```python
from build123d import *

# Parameters (mm, degrees)
BOSS_EXTRUDE1_DEPTH     = 16
F_8_0MM_DOWEL_HOLE1_D   = 8
CIRPATTERN2_COUNT       = 5
CIRPATTERN2_ANGLE       = 180
MIRROR2_COPY_1_D        = 8
MIRROR2_COPY_2_D        = 8
MIRROR2_COPY_3_D        = 8
MIRROR2_COPY_4_D        = 8
LPATTERN1_COUNT         = 3
LPATTERN1_PITCH         = 74
MIRROR3_COPY_1_D        = 8
MIRROR3_COPY_2_D        = 8
MIRROR3_COPY_3_D        = 8
SKETCH13_R              = 4
SKETCH13_R_2            = 10
BOSS_EXTRUDE2_DEPTH     = 16
BOSS_EXTRUDE3_DEPTH     = 26
SKETCH16_W              = 10
SKETCH16_H              = 10
BOSS_EXTRUDE5_DEPTH     = 5
M10X1_25_TAPPED_HOLE1_D = 8.8
SKETCH19_R              = 16
CUT_EXTRUDE1_DEPTH      = 32


with BuildPart() as part:
    # Sketch1 → Boss-Extrude1 (new body)
    with BuildSketch(Plane(origin=(0, 0, 0), x_dir=(1, 0, 0), z_dir=(0, 1, 0))):
        with BuildLine():
            Line((-110, 110), (110, 110))
            ThreePointArc((110, 110), (220, 0), (110, -110))
            Line((110, -110), (-110, -110))
            ThreePointArc((-110, -110), (-220, 0), (-110, 110))
        make_face()
        with BuildLine():
            Line((-110, 90), (110, 90))
            ThreePointArc((110, 90), (200, 0), (110, -90))
            Line((110, -90), (-110, -90))
            ThreePointArc((-110, -90), (-200, 0), (-110, 90))
        make_face(mode=Mode.SUBTRACT)
    extrude(amount=BOSS_EXTRUDE1_DEPTH)

    # Ø8.0mm Dowel Hole1 (through all)
    with Locations(Plane(origin=(-110, 16, -100), x_dir=(0, 0, 1), z_dir=(0, 1, 0))):
        with Locations((0, 0)):
            f_8_0mm_dowel_hole1 = Hole(F_8_0MM_DOWEL_HOLE1_D / 2)

    # CirPattern2: Ø8.0mm Dowel Hole1 ×5 about axis
    cirpattern2_axis = Axis((-110, 0, 0), (0, 1, 0))
    for i in range(1, CIRPATTERN2_COUNT):
        add(f_8_0mm_dowel_hole1.rotate(cirpattern2_axis, i * CIRPATTERN2_ANGLE / (CIRPATTERN2_COUNT - 1)), mode=Mode.SUBTRACT)

    # Mirror2: Ø8.0mm Dowel Hole1 across plane
    add(f_8_0mm_dowel_hole1.mirror(Plane(origin=(0, 0, 0), x_dir=(0, 0, 1), z_dir=(1, 0, 0))), mode=Mode.SUBTRACT)

    # Mirror2 copy 1 (through all)
    with Locations(Plane(origin=(180.710678119, 16, -70.710678119), x_dir=(-0.707106781, 0, 0.707106781), z_dir=(0, 1, 0))):
        with Locations((0, 0)):
            Hole(MIRROR2_COPY_1_D / 2)

    # Mirror2 copy 2 (through all)
    with Locations(Plane(origin=(210, 16, 0), x_dir=(-1, 0, 0), z_dir=(0, 1, 0))):
        with Locations((0, 0)):
            Hole(MIRROR2_COPY_2_D / 2)

    # Mirror2 copy 3 (through all)
    with Locations(Plane(origin=(180.710678119, 16, 70.710678119), x_dir=(-0.707106781, 0, -0.707106781), z_dir=(0, 1, 0))):
        with Locations((0, 0)):
            Hole(MIRROR2_COPY_3_D / 2)

    # Mirror2 copy 4 (through all)
    with Locations(Plane(origin=(110, 16, 100), x_dir=(0, 0, -1), z_dir=(0, 1, 0))):
        with Locations((0, 0)):
            Hole(MIRROR2_COPY_4_D / 2)

    # LPattern1: Ø8.0mm Dowel Hole1 ×3
    with Locations(*[(i * LPATTERN1_PITCH, 0, 0) for i in range(1, LPATTERN1_COUNT)]):
        add(f_8_0mm_dowel_hole1, mode=Mode.SUBTRACT)

    # Mirror3 copy 1 (through all)
    with Locations(Plane(origin=(-36, 16, 100), x_dir=(0, 0, -1), z_dir=(0, 1, 0))):
        with Locations((0, 0)):
            Hole(MIRROR3_COPY_1_D / 2)

    # Mirror3 copy 2 (through all)
    with Locations(Plane(origin=(38, 16, 100), x_dir=(0, 0, -1), z_dir=(0, 1, 0))):
        with Locations((0, 0)):
            Hole(MIRROR3_COPY_2_D / 2)

    # Mirror3 copy 3 (through all)
    with Locations(Plane(origin=(-110, 16, 100), x_dir=(0, 0, -1), z_dir=(0, 1, 0))):
        with Locations((0, 0)):
            Hole(MIRROR3_COPY_3_D / 2)

    # Sketch13 → Boss-Extrude2 (add)
    with BuildSketch(Plane(origin=(0, 0, 0), x_dir=(1, 0, 0), z_dir=(0, 1, 0))):
        with BuildLine():
            Line((-110, -110), (110, -110))
            ThreePointArc((110, -110), (220, 0), (110, 110))
            Line((110, 110), (-110, 110))
            ThreePointArc((-110, 110), (-220, 0), (-110, -110))
        make_face()
        with Locations((38, -100)):
            Circle(SKETCH13_R, mode=Mode.SUBTRACT)
        with Locations((-110, 100)):
            Circle(SKETCH13_R, mode=Mode.SUBTRACT)
        with Locations((-180.710678119, 70.710678119)):
            Circle(SKETCH13_R, mode=Mode.SUBTRACT)
        with Locations((-210, 0)):
            Circle(SKETCH13_R, mode=Mode.SUBTRACT)
        with Locations((-180.710678119, -70.710678119)):
            Circle(SKETCH13_R, mode=Mode.SUBTRACT)
        with Locations((-110, -100)):
            Circle(SKETCH13_R, mode=Mode.SUBTRACT)
        with Locations((110, 100)):
            Circle(SKETCH13_R, mode=Mode.SUBTRACT)
        with Locations((180.710678119, 70.710678119)):
            Circle(SKETCH13_R, mode=Mode.SUBTRACT)
        with Locations((210, 0)):
            Circle(SKETCH13_R, mode=Mode.SUBTRACT)
        with Locations((180.710678119, -70.710678119)):
            Circle(SKETCH13_R, mode=Mode.SUBTRACT)
        with Locations((110, -100)):
            Circle(SKETCH13_R, mode=Mode.SUBTRACT)
        with Locations((-36, 100)):
            Circle(SKETCH13_R, mode=Mode.SUBTRACT)
        with Locations((38, 100)):
            Circle(SKETCH13_R, mode=Mode.SUBTRACT)
        with Locations((-36, -100)):
            Circle(SKETCH13_R, mode=Mode.SUBTRACT)
        with Locations((-165, -50)):
            Circle(SKETCH13_R_2, mode=Mode.SUBTRACT)
        with Locations((-165, 50)):
            Circle(SKETCH13_R_2, mode=Mode.SUBTRACT)
    extrude(amount=BOSS_EXTRUDE2_DEPTH)

    # Sketch15 → Boss-Extrude3 (add)
    with BuildSketch(Plane(origin=(0, 0, 0), x_dir=(1, 0, 0), z_dir=(0, 1, 0))):
        with BuildLine():
            ThreePointArc((-130, 70), (-124.142135624, 84.142135624), (-110, 90))
            Line((-110, 90), (110, 90))
            Line((110, 90), (110, -90))
            Line((110, -90), (-110, -90))
            ThreePointArc((-110, -90), (-124.142135624, -84.142135624), (-130, -70))
            Line((-130, -70), (-130, 70))
        make_face()
        with BuildLine():
            ThreePointArc((110, 90), (200, 0), (110, -90))
            Line((110, -90), (110, 90))
        make_face()
    extrude(amount=BOSS_EXTRUDE3_DEPTH)

    # Sketch16 → Boss-Extrude5 (add)
    with BuildSketch(Plane(origin=(0, 26, 0), x_dir=(1, 0, 0), z_dir=(0, 1, 0))):
        with BuildLine():
            Line((-62.14, 29.580398915), (-62.14, 5))
            Line((-62.14, 5), (-52.14, 5))
            Line((-52.14, 5), (-52.14, 29.580398915))
            ThreePointArc((-52.14, 29.580398915), (-57.14, 30), (-62.14, 29.580398915))
        make_face()
        with BuildLine():
            Line((-52.14, 90), (-62.14, 90))
            Line((-62.14, 90), (-62.14, 29.580398915))
            ThreePointArc((-62.14, 29.580398915), (-57.14, 30), (-52.14, 29.580398915))
            Line((-52.14, 29.580398915), (-52.14, 90))
        make_face()
        with BuildLine():
            Line((-52.14, 29.580398915), (-52.14, 5))
            Line((-52.14, 5), (-27.559601085, 5))
            ThreePointArc((-27.559601085, 5), (-35.926796564, 21.213203436), (-52.14, 29.580398915))
        make_face()
        with BuildLine():
            Line((-27.559601085, 5), (-52.14, 5))
            Line((-52.14, 5), (-52.14, -5))
            Line((-52.14, -5), (-27.559601085, -5))
            ThreePointArc((-27.559601085, -5), (-27.245084316, -2.508787808), (-27.14, 0))
            ThreePointArc((-27.14, 0), (-27.245084316, 2.508787808), (-27.559601085, 5))
        make_face()
        with Locations((-57.14, 0)):
            Rectangle(SKETCH16_W, SKETCH16_H)
        with BuildLine():
            Line((-52.14, -5), (-62.14, -5))
            Line((-62.14, -5), (-62.14, -29.580398915))
            ThreePointArc((-62.14, -29.580398915), (-57.14, -30), (-52.14, -29.580398915))
            Line((-52.14, -29.580398915), (-52.14, -5))
        make_face()
        with BuildLine():
            Line((-62.14, 5), (-86.720398915, 5))
            ThreePointArc((-86.720398915, 5), (-87.14, 0), (-86.720398915, -5))
            Line((-86.720398915, -5), (-62.14, -5))
            Line((-62.14, -5), (-62.14, 5))
        make_face()
        with BuildLine():
            ThreePointArc((-62.14, 29.580398915), (-78.353203436, 21.213203436), (-86.720398915, 5))
            Line((-86.720398915, 5), (-62.14, 5))
            Line((-62.14, 5), (-62.14, 29.580398915))
        make_face()
        with BuildLine():
            Line((-62.14, -5), (-86.720398915, -5))
            ThreePointArc((-86.720398915, -5), (-78.353203436, -21.213203436), (-62.14, -29.580398915))
            Line((-62.14, -29.580398915), (-62.14, -5))
        make_face()
        with BuildLine():
            Line((-27.559601085, -5), (-52.14, -5))
            Line((-52.14, -5), (-52.14, -29.580398915))
            ThreePointArc((-52.14, -29.580398915), (-35.926796564, -21.213203436), (-27.559601085, -5))
        make_face()
        with BuildLine():
            Line((26.43, 5), (-27.559601085, 5))
            ThreePointArc((-27.559601085, 5), (-27.245084316, 2.508787808), (-27.14, 0))
            ThreePointArc((-27.14, 0), (-27.245084316, -2.508787808), (-27.559601085, -5))
            Line((-27.559601085, -5), (26.43, -5))
            Line((26.43, -5), (80.419601085, -5))
            ThreePointArc((80.419601085, -5), (80, 0), (80.419601085, 5))
            Line((80.419601085, 5), (26.43, 5))
        make_face()
        with BuildLine():
            Line((-86.720398915, 5), (-130, 5))
            Line((-130, 5), (-130, -5))
            Line((-130, -5), (-86.720398915, -5))
            ThreePointArc((-86.720398915, -5), (-87.14, 0), (-86.720398915, 5))
        make_face()
        with BuildLine():
            ThreePointArc((-52.14, -29.580398915), (-57.14, -30), (-62.14, -29.580398915))
            Line((-62.14, -29.580398915), (-62.14, -90))
            Line((-62.14, -90), (-52.14, -90))
            Line((-52.14, -90), (-52.14, -29.580398915))
        make_face()
        with BuildLine():
            ThreePointArc((139.580398915, 5), (131.213203436, 21.213203436), (115, 29.580398915))
            Line((115, 29.580398915), (115, 5))
            Line((115, 5), (139.580398915, 5))
        make_face()
        with BuildLine():
            ThreePointArc((115, 29.580398915), (110, 30), (105, 29.580398915))
            Line((105, 29.580398915), (105, 5))
            Line((105, 5), (115, 5))
            Line((115, 5), (115, 29.580398915))
        make_face()
        with BuildLine():
            Line((105, 5), (105, 29.580398915))
            ThreePointArc((105, 29.580398915), (88.786796564, 21.213203436), (80.419601085, 5))
            Line((80.419601085, 5), (105, 5))
        make_face()
        with BuildLine():
            Line((105, -5), (105, 5))
            Line((105, 5), (80.419601085, 5))
            ThreePointArc((80.419601085, 5), (80, 0), (80.419601085, -5))
            Line((80.419601085, -5), (105, -5))
        make_face()
        with Locations((110, 0)):
            Rectangle(SKETCH16_W, SKETCH16_H)
        with BuildLine():
            Line((139.580398915, 5), (115, 5))
            Line((115, 5), (115, -5))
            Line((115, -5), (139.580398915, -5))
            ThreePointArc((139.580398915, -5), (139.894915684, -2.508787808), (140, 0))
            ThreePointArc((140, 0), (139.894915684, 2.508787808), (139.580398915, 5))
        make_face()
        with BuildLine():
            Line((139.580398915, -5), (115, -5))
            Line((115, -5), (115, -29.580398915))
            ThreePointArc((115, -29.580398915), (131.213203436, -21.213203436), (139.580398915, -5))
        make_face()
        with BuildLine():
            Line((115, -5), (105, -5))
            Line((105, -5), (105, -29.580398915))
            ThreePointArc((105, -29.580398915), (110, -30), (115, -29.580398915))
            Line((115, -29.580398915), (115, -5))
        make_face()
        with BuildLine():
            Line((105, -29.580398915), (105, -5))
            Line((105, -5), (80.419601085, -5))
            ThreePointArc((80.419601085, -5), (88.786796564, -21.213203436), (105, -29.580398915))
        make_face()
        with BuildLine():
            ThreePointArc((199.861003778, -5), (200, 0), (199.861003778, 5))
            Line((199.861003778, 5), (139.580398915, 5))
            ThreePointArc((139.580398915, 5), (139.894915684, 2.508787808), (140, 0))
            ThreePointArc((140, 0), (139.894915684, -2.508787808), (139.580398915, -5))
            Line((139.580398915, -5), (199.861003778, -5))
        make_face()
        with BuildLine():
            Line((110, 90), (105, 90))
            Line((105, 90), (105, 29.580398915))
            ThreePointArc((105, 29.580398915), (110, 30), (115, 29.580398915))
            Line((115, 29.580398915), (115, 89.861003778))
            ThreePointArc((115, 89.861003778), (112.500965811, 89.965244234), (110, 90))
        make_face()
        with BuildLine():
            Line((105, -29.580398915), (105, -90))
            Line((105, -90), (110, -90))
            ThreePointArc((110, -90), (112.500965811, -89.965244234), (115, -89.861003778))
            Line((115, -89.861003778), (115, -29.580398915))
            ThreePointArc((115, -29.580398915), (110, -30), (105, -29.580398915))
        make_face()
    extrude(amount=BOSS_EXTRUDE5_DEPTH)

    # M10x1.25 Tapped Hole1 (through all)
    with Locations(Plane(origin=(-56.866813058, 31, 0), x_dir=(0, 0, 1), z_dir=(0, 1, 0))):
        with Locations((0, 0)):
            Hole(M10X1_25_TAPPED_HOLE1_D / 2)

    # Sketch19 → Cut-Extrude1 (cut, through all)
    with BuildSketch(Plane(origin=(0, 31, 0), x_dir=(1, 0, 0), z_dir=(0, 1, 0))):
        with Locations((110, 0)):
            Circle(SKETCH19_R)
    extrude(amount=-CUT_EXTRUDE1_DEPTH, mode=Mode.SUBTRACT)


solid = part.part
```
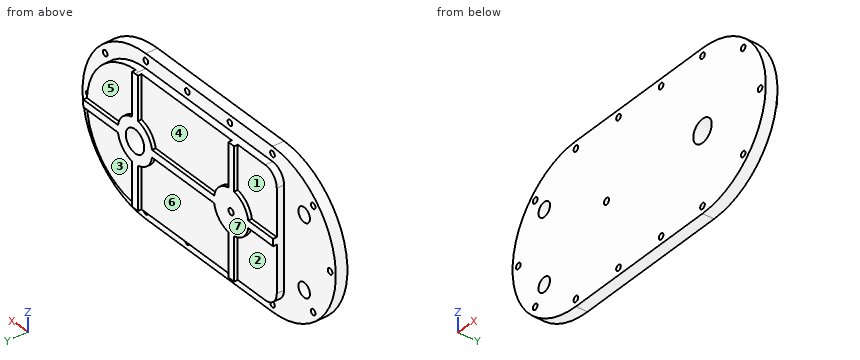
Geometry check sheet. Reference: the model listing, model coordinates, mm. Face numbers are marked on the shaded views. A direction names the side the tool comes from. Round coordinates to 2 decimals unless told otherwise and drop trailing zeros. Order: outer loops, then holes, each group sorted by start corner. A loop starts at its lowest first (then second) coordinate and runs counter-clockwise, first axis right, second up. Notation, with made-up numbers: (39, 33.5) -> (75, 33.5) arc R24 cw to (75, 47.5) -> close; hole circle Ø10 at (67.5, 7.25). An arc over 180 degrees is marked (long way). Return JSON: item names as keys, results as strings. Group by question number.
Q1. Section check C-C, the plane x = -210. Record the boundary of the cut face in (y, z).
Q2. Material ranges on probe 1 along Z at (x, y) = (-36, 4.5); probe 2 along Z at (x, y) = (110, 8.25); probe 3 along X at (y, z) = (4, 100), recorded low to high. Write a range as from..to.
Q3. Section check A-A, the plane z = 0. Record the boundary of the cut face in (x, y), plus the area to 3 significant figures.
Q4. Section check D-D, the plane z = -54. Record the boundary of the cut face in (x, y).
Q5. Release check for a two-part mould opening along X. For the marked faces 6 and 7 record: released by +X, released by -X, zero draft, split by the parting line, or undercut.
Q6. Section check B-B, the plane x = 38. Record the boundary of the cut face in (y, z), plus the area to 3 significant figures.
Q7. Tool access check on the marked faces 1, 2, 3, 4 and 5. Record the directions out of +Z, -Z, +X, -X, +Y, -Y that give a thin tool (end or side, any length) a straight path to the whole face; none if there is none.
Q8. Gauge pin test, flat ends, axial feed: pin 1 (1.5 mm diameter, centred on y = 18, z = -6, fed in from +X); pin 2 (5 mm diameter, centred on y = 7, z = 64.5, fed in from +X); pin 3 (2.5 mm diameter, centred on x = 156.5, y = 28.5, fed in from -Z). Record the tip position at first contact, or that the pin passes through.
Numbers:
{
 "1": {"outline": "(0, -45.83) -> (16, -45.83) -> (16, -4) -> (0, -4) -> close; (0, 4) -> (16, 4) -> (16, 45.83) -> (0, 45.83) -> close"},
 "2": {"probe 1": "-110..-104, -96..96, 104..110", "probe 2": "-110..-104, -96..-16, 16..96, 104..110", "probe 3": "-155.83..-114, -106..-40, -32..34, 42..106, 114..155.83"},
 "3": {"outline": "(-220, 0) -> (-214, 0) -> (-214, 16) -> (-220, 16) -> close; (-206, 0) -> (-61.27, 0) -> (-61.27, 31) -> (-130, 31) -> (-130, 16) -> (-206, 16) -> close; (-52.47, 0) -> (94, 0) -> (94, 31) -> (-52.47, 31) -> close; (126, 0) -> (206, 0) -> (206, 16) -> (200, 16) -> (200, 31) -> (126, 31) -> close; (214, 0) -> (220, 0) -> (220, 16) -> (214, 16) -> close", "area": "10,500 mm^2"},
 "4": {"outline": "(-205.83, 0) -> (-174.17, 0) -> (-174.17, 16) -> (-205.83, 16) -> close; (-155.83, 0) -> (205.83, 0) -> (205.83, 16) -> (182, 16) -> (182, 26) -> (115, 26) -> (115, 31) -> (105, 31) -> (105, 26) -> (-52.14, 26) -> (-52.14, 31) -> (-62.14, 31) -> (-62.14, 26) -> (-130, 26) -> (-130, 16) -> (-155.83, 16) -> close"},
 "5": {"face 6": "undercut", "face 7": "zero draft"},
 "6": {"outline": "(0, -110) -> (16, -110) -> (16, -104) -> (0, -104) -> close; (0, -96) -> (16, -96) -> (16, -90) -> (26, -90) -> (26, -5) -> (31, -5) -> (31, 5) -> (26, 5) -> (26, 90) -> (16, 90) -> (16, 96) -> (0, 96) -> close; (0, 104) -> (16, 104) -> (16, 110) -> (0, 110) -> close", "area": "5,110 mm^2"},
 "7": {"face 1": "+Z, -X, +Y", "face 2": "-Z, -X, +Y", "face 3": "-Z, +X, +Y", "face 4": "+Z, +Y", "face 5": "+Z, +X, +Y"},
 "8": {"pin 1": "x = 199.85", "pin 2": "x = 200.86", "pin 3": "z = -5"}
}
